```python
from build123d import *

# Parameters (mm, degrees)
F0_W     = 100
F0_H     = 50
F1_DEPTH = 2.5


with BuildPart() as f1:
    # F0 (on Front) → F1 (new body, symmetric)
    with BuildSketch(Plane.XZ):
        Rectangle(F0_W, F0_H)
        with BuildLine():
            ThreePointArc((10.375, 0), (2.835445, -9.980024), (-8.825169, -5.455))
            Line((-8.825169, -5.455), (-8.825169, 0))
            Line((-8.825169, 0), (-8.825169, 5.455))
            ThreePointArc((-8.825169, 5.455), (2.835445, 9.980024), (10.375, 0))
        make_face(mode=Mode.SUBTRACT)
    extrude(amount=F1_DEPTH, both=True)


solid = f1.part
```
Here's how the part is built. I have some questions about the finished solid (model axes, mm). A direction names the side the tool comes from. Give positions to 0.01 mm unless a question says otherwise; leave off trailing zeros. Loops run counter-clockwise (first coordinate to the right, second up) from the corner with the lowest first, then second, coordinate; pieces in that order, holes last. Notation, with made-up numbers: M 59.25,75 L 108.25,75 A28 cw 108.25,93 Z; hole C 24.5,79 d3. An arc over 180 degrees is marked long. Return JSON: item names as keys, results as strings.
Item 1: Imagine slicing it at A-A on z = 0. List the corners of the cut face in (x, y) for me (3 decimals).
A:
{"outline": "M -50,-2.5 L -8.825,-2.5 L -8.825,2.5 L -50,2.5 Z; M 10.375,-2.5 L 50,-2.5 L 50,2.5 L 10.375,2.5 Z"}
Item 2: Imagine slicing it at C-C on y = -0.15. List the corners of the cut face in (x, z) for me (3 decimals).
A:
{"outline": "M -50,-25 L 50,-25 L 50,25 L -50,25 Z; hole M -8.825,-5.455 A10.375 ccw long -8.825,5.455 Z"}
Item 3: Thinking about a two-plate mould opening in X: for faces 3 (the cylindrical face through (10.37, -0.04, 0.38)), 4 (the flat face through (-1, 2.5, 11)), 5 (the flat face through (-50, 0, 0)), which applies, released by +X, released by -X, zero draft, split by the parting line, or undercut?
A:
{"face 3": "undercut", "face 4": "zero draft", "face 5": "released by -X"}
Item 4: On a 3-axis mill with a long thin cutter (end or side, diameter ignored), from which of +Z, -Z, +X, -X, +Y, -Y can I reach the whole of each face in a straight line? I mean faces 1 (the flat face through (-8.825, 0, 0)), 2 (the flat face through (-1, 0, -25)). Say none if no direction works.
A:
{"face 1": "+Y, -Y", "face 2": "-Z, +X, -X, +Y, -Y"}
Item 5: Imagine slicing it at B-B on x = 0. List the corners of the cut face in (y, z) for me (3 decimals), then the cut area to 3 significant figures.
A:
{"outline": "M -2.5,-25 L 2.5,-25 L 2.5,-10.375 L -2.5,-10.375 Z; M -2.5,10.375 L 2.5,10.375 L 2.5,25 L -2.5,25 Z", "area": "146 mm^2"}
Item 6: Please list where these lines run through material, in increasing order: line 1 (Z direction, x = 0, y = -0.6) (3 decimals); line 2 (X direction, y = 1.1, z = 0) (3 decimals); line 3 (X direction, y = 0.45, z = -4).
A:
{"line 1": "z = -25 to -10.375, 10.375 to 25", "line 2": "x = -50 to -8.825, 10.375 to 50", "line 3": "x = -50 to -8.83, 9.57 to 50"}
